The model under review builds one solid part; all positions refer to its coordinate system, in mm. A direction names the side the tool comes from. Round coordinates to 2 decimals unless told otherwise and drop trailing zeros. Loops run counter-clockwise (first coordinate to the right, second up) from the corner with the lowest first, then second, coordinate; pieces in that order, holes last. Notation, with made-up numbers: M 4,80 L 36,80 A17 cw 36,97 Z; hole C 42.5,78.5 d7. An arc over 180 degrees is marked long. Answer as a JSON object with one key per item and string values. Group by question number.
Item 1: Consider section B-B (y = 0). Give the boundary of the cut face in (x, z), and give its area (3 significant figures).
Item 2: To check wall thickness, follow line 1 (X direction, y = 0, z = -26.5); line 2 (Y direction, x = -8, z = 0); line 3 (Y direction, x = 0.25, z = -2.5). State the ranges of each line that lie inside material, in increasing order.
Item 3: Consider section C-C (z = 3.5). Give the boundary of the cut face in (x, y), and give its area (3 significant figures).
Item 4: Consider section D-D (z = -35). Give the boundary of the cut face in (x, y).
Item 5: Insertion check: P1, Ø2, axis at x = 3, z = 0.5, coming from the +Y side; P2, Ø3, axis at y = 4.5, z = 8.5, coming from the -X side; P3, Ø4.5, axis at x = -7.5, z = 4, coming from the +Y side. Each pin has a flat end and moves straight along its axis. Give the tip position at first contact, or say it passes through.
Item 6: Consider section A-A (x = 0). Give the boundary of the cut face in (y, z).
Item 7: The part is to be moulded in two halves that separate along Y. For faces 3 (the face through (-3.649, 7.296, 30.784)), 4 (the face through (0.2, -9.2, 44.8)), 5 (the face through (3.075, -4.01, -29.283)), say which applies: +Y half, -Y half, draft (parallel to the pull), parting line (faces both ways), or undercut.
Item 8: Tool access review of faces 1 (the face through (0, 6, 14)), 2 (the face through (4, -4, -45)): name each direction out of +Z, -Z, +X, -X, +Y, -Y from which nothing blocks a thin tool from reaching the whole face with its end or side.
Autodesk Inventor part; units mm, degrees
ref_plane "YZ Plane" through (0, 0, 0) normal (1, 0, 0) x (0, 1, 0)
ref_plane "XY Plane" through (0, 0, 0) normal (0, 0, 1) x (1, 0, 0)
sketch "Sketch1" plane through (0, 0, 0) normal (0, 0, 1) x (1, 0, 0)
  circle A0 centre (0, 0) radius 10
  dimension "d0" = 20
extrude "Extrusion1" add sketch "Sketch1" along normal mid plane 90
sketch "Sketch2" plane through (0, 0, 45) normal (0, 0, 1) x (1, 0, 0)
  circle A0 centre (0, 0) radius 6
  line L0 (-10, -2.5) -> (10, -2.5)
  line L1 (10, -2.5) -> (10, 2.5)
  line L2 (10, 2.5) -> (-10, 2.5)
  line L3 (-10, 2.5) -> (-10, -2.5)
  point P0 (-10, 0)
  point P1 (10, 0)
  dimension "d3" = 12
  dimension "d4" = 5
  dimension "d5" = 2.5
  dimension "d6" = 20
  dimension "d7" = 10
extrude "Extrusion2" cut sketch "Sketch2" against normal blind 59
chamfer "Chamfer1" distance 1 angle 45 2 edges at (0, -10, 45) (0, 10, 45)
chamfer "Chamfer2" distance 1.5 distance2 4 1 edges at (0, 6, 45) measured on face at (-7.3096, 3.1466, 45)
chamfer "Chamfer3" distance 1.5 distance2 4 1 edges at (0, -6, 45) measured on face at (-7.3096, -3.1466, 45)
chamfer "Chamfer4" distance 4 distance2 2 1 edges at (-10, 0, -14) measured on face at (8.4358, 5.37, -15.3333)
chamfer "Chamfer5" distance 4 distance2 2 2 edges at (9.9203, 1.26, -14) (9.9203, -1.26, -14) measured on face at (8.4358, 5.37, -15.3333)
chamfer "Chamfer6" distance 1 angle 45 1 edges at (-10, 0, -45)
sketch "Sketch3" plane through (0, 0, -45) normal (0, 0, -1) x (-1, 0, 0)
  circle A0 centre (0, 0) radius 9
hole "Hole1" at (0, 0, -45) direction (0, 0, 1) diameter 10.106 depth 45
sketch "Sketch4" plane through (0, 0, 0) normal (0, 1, 0) x (-1, 0, 0)
  line L0 (0, -9) -> (0, 54)
  circle A0 centre (0, 32.297) radius 3.95
  line L1 (-8.6458, 45) -> (8.6458, 45)
  point P0 (0, 0)
  dimension "d35" = 12.703
  dimension "d36" = 7.9
extrude "Extrusion3" cut sketch "Sketch4" along normal through all both and the other way through all
properties part number "201-02" material "Acetal Resin, Black"
Geometry results:
{
 "1": {"outline": "M -10,-44 L -9,-45 L -5.05,-45 L -5.05,-14 L -8,-14 L -10,-18 Z; M 5.05,-45 L 9,-45 L 10,-44 L 10,-18 L 8,-14 L 5.05,-14 Z", "area": "298 mm^2"},
 "2": {"line 1": "x = -10 to -5.05, 5.05 to 10", "line 2": "y = -6 to -2.5, 2.5 to 6", "line 3": "y = -10 to -5.99, 5.99 to 10"},
 "3": {"outline": "M -9.68,-2.5 A10 ccw 9.68,-2.5 L 5.45,-2.5 A6 cw -5.45,-2.5 Z; M -9.68,2.5 L -5.45,2.5 A6 cw 5.45,2.5 L 9.68,2.5 A10 ccw Z", "area": "160 mm^2"},
 "4": {"outline": "C 0,0 d20; hole C 0,0 d10.11"},
 "5": {"P1": "stops at y = 9.8", "P2": "stops at x = -9.54", "P3": "stops at y = 8.51"},
 "6": {"outline": "M -10,-44 L -9,-45 L -5.05,-45 L -5.05,-14 L -6,-14 L -6,28.35 L -10,28.35 Z; M -10,36.25 L -6,36.25 L -6,41 L -7.5,45 L -9,45 L -10,44 Z; M 5.05,-45 L 9,-45 L 10,-44 L 10,28.35 L 6,28.35 L 6,-14 L 5.05,-14 Z; M 6,36.25 L 10,36.25 L 10,44 L 9,45 L 7.5,45 L 6,41 Z"},
 "7": {"face 3": "draft", "face 4": "-Y half", "face 5": "undercut"},
 "8": {"face 1": "+Z", "face 2": "-Z, +X, -X, +Y, -Y"}
}
